Can you work these out from the model? Positions are in its coordinate system, mm. Face numbers are marked on the shaded views. A direction names the side the tool comes from. Coordinates: 2 decimals unless noted, no trailing zeros. Order: outer loops, then holes, each group sorted by start corner. A loop starts at its lowest first (then second) coordinate and runs counter-clockwise, first axis right, second up. Notation, with made-up numbers: (85, 4.25) -> (119, 4.25) arc R22 ccw to (119, 32.25) -> close; hole circle Ø11 at (78, 64). An arc over 180 degrees is marked (long way). Return JSON: item names as keys, results as strings. Group by question number.
1) If we section it at C-C, the plane y = 45.3: Please give me the cut outline in (x, z), then the cut area to 3 significant figures.
2) If we section it at B-B, the plane y = 30: Please give me the cut outline in (x, z).
3) For the marked faces 1 and 2, which set-ups out of +Z, -Z, +X, -X, +Y, -Y let a thin tool reach every point of the face, with its end or its side?
4) If we section it at A-A, the plane z = 0: Please give me the cut outline in (x, y), then the cut area to 3 significant figures.
5) If I drill on probe 1 along X at (y, z) = (0.9, -12.7); probe 2 along X at (y, z) = (29.5, -12.5), over which ranges is the centre line in solid material (lowest first)? Write a range as from..to.
6) For pin 1 (10 mm diameter, centred on x = 11.5, z = 14.5, fed in from +Y); pin 2 (6 mm diameter, centred on y = 11, z = -17.5, fed in from +X); pin 3 (12 mm diameter, centred on x = 41, y = 11.5, fed in from +Z), each with a flat end and sliding along its axis, tell me the tip position at first contact or that it passes through.
7) If we section it at D-D, the plane z = 18.25: Please give me the cut outline in (x, y).
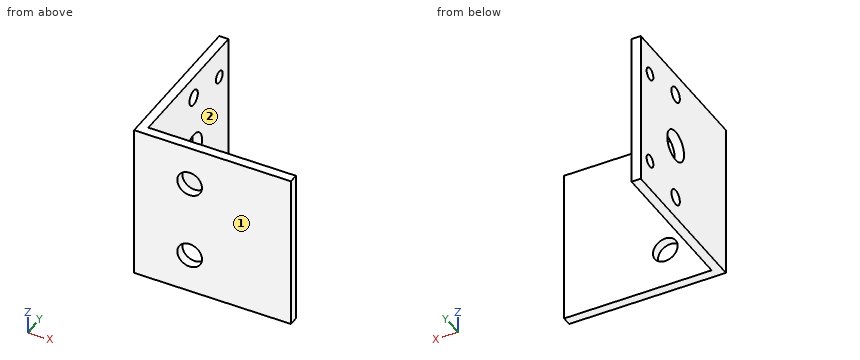
from build123d import *

# Parameters (mm, degrees)
EXTRUDE_THIN1_DEPTH = 25.4
CUT_EXTRUDE1_REACH  = 78.2
SKETCH2_R           = 2.5
SKETCH2_R_2         = 5
CUT_EXTRUDE2_REACH  = 78.2
SKETCH3_R           = 4
CUT_EXTRUDE3_REACH  = 78.2
SKETCH4_R           = 2


with BuildPart() as part:
    # Sketch1 → Extrude-Thin1 (new, symmetric)
    with BuildSketch(Plane.XY):
        Polygon((50.8, 0), (0, 0), (0, 50.8), (3, 50.8), (3, 3), (50.8, 3), align=None)
    extrude(amount=EXTRUDE_THIN1_DEPTH, both=True)

    # Sketch2 → Cut-Extrude1 (cut, up to next)
    with BuildSketch(Plane.ZY, mode=Mode.PRIVATE) as cut_extrude1_sk1:
        with Locations((-18.25, 30)):
            Circle(SKETCH2_R)
    cut_extrude1_tool1 = extrude(cut_extrude1_sk1.sketch, amount=-CUT_EXTRUDE1_REACH, mode=Mode.PRIVATE) & part.part
    # Sketch2 → Cut-Extrude1 (cut, up to next)
    with BuildSketch(Plane.ZY, mode=Mode.PRIVATE) as cut_extrude1_sk2:
        with Locations((18.25, 30)):
            Circle(SKETCH2_R)
    cut_extrude1_tool2 = extrude(cut_extrude1_sk2.sketch, amount=-CUT_EXTRUDE1_REACH, mode=Mode.PRIVATE) & part.part
    # Sketch2 → Cut-Extrude1 (cut, up to next)
    with BuildSketch(Plane.ZY, mode=Mode.PRIVATE) as cut_extrude1_sk3:
        with Locations((0, 30)):
            Circle(SKETCH2_R_2)
    cut_extrude1_tool3 = extrude(cut_extrude1_sk3.sketch, amount=-CUT_EXTRUDE1_REACH, mode=Mode.PRIVATE) & part.part
    add(cut_extrude1_tool1.solids().sort_by_distance((0, 30, -18.25))[0], mode=Mode.SUBTRACT)
    add(cut_extrude1_tool2.solids().sort_by_distance((0, 30, 18.25))[0], mode=Mode.SUBTRACT)
    add(cut_extrude1_tool3.solids().sort_by_distance((0, 30, 0))[0], mode=Mode.SUBTRACT)

    # Sketch3 → Cut-Extrude2 (cut, up to next)
    with BuildSketch(Plane.XZ, mode=Mode.PRIVATE) as cut_extrude2_sk1:
        with Locations(Location((18, 12.7, 0), (0, 0, 270))):
            Circle(SKETCH3_R)
    cut_extrude2_tool1 = extrude(cut_extrude2_sk1.sketch, amount=-CUT_EXTRUDE2_REACH, mode=Mode.PRIVATE) & part.part
    # Sketch3 → Cut-Extrude2 (cut, up to next)
    with BuildSketch(Plane.XZ, mode=Mode.PRIVATE) as cut_extrude2_sk2:
        with Locations(Location((18, -12.7, 0), (0, 0, 270))):
            Circle(SKETCH3_R)
    cut_extrude2_tool2 = extrude(cut_extrude2_sk2.sketch, amount=-CUT_EXTRUDE2_REACH, mode=Mode.PRIVATE) & part.part
    add(cut_extrude2_tool1.solids().sort_by_distance((18, 0, 12.7))[0], mode=Mode.SUBTRACT)
    add(cut_extrude2_tool2.solids().sort_by_distance((18, 0, -12.7))[0], mode=Mode.SUBTRACT)

    # Sketch4 → Cut-Extrude3 (cut, up to next)
    with BuildSketch(Plane.ZY, mode=Mode.PRIVATE) as cut_extrude3_sk1:
        with Locations((-15.5, 45.3)):
            Circle(SKETCH4_R)
    cut_extrude3_tool1 = extrude(cut_extrude3_sk1.sketch, amount=-CUT_EXTRUDE3_REACH, mode=Mode.PRIVATE) & part.part
    # Sketch4 → Cut-Extrude3 (cut, up to next)
    with BuildSketch(Plane.ZY, mode=Mode.PRIVATE) as cut_extrude3_sk2:
        with Locations((15.5, 45.3)):
            Circle(SKETCH4_R)
    cut_extrude3_tool2 = extrude(cut_extrude3_sk2.sketch, amount=-CUT_EXTRUDE3_REACH, mode=Mode.PRIVATE) & part.part
    add(cut_extrude3_tool1.solids().sort_by_distance((0, 45.3, -15.5))[0], mode=Mode.SUBTRACT)
    add(cut_extrude3_tool2.solids().sort_by_distance((0, 45.3, 15.5))[0], mode=Mode.SUBTRACT)


solid = part.part
Result sheet:
{
 "1": {"outline": "(0, -25.4) -> (3, -25.4) -> (3, -17.5) -> (0, -17.5) -> close; (0, -13.5) -> (3, -13.5) -> (3, 13.5) -> (0, 13.5) -> close; (0, 17.5) -> (3, 17.5) -> (3, 25.4) -> (0, 25.4) -> close", "area": "128 mm2"},
 "2": {"outline": "(0, -25.4) -> (3, -25.4) -> (3, -20.75) -> (0, -20.75) -> close; (0, -15.75) -> (3, -15.75) -> (3, -5) -> (0, -5) -> close; (0, 5) -> (3, 5) -> (3, 15.75) -> (0, 15.75) -> close; (0, 20.75) -> (3, 20.75) -> (3, 25.4) -> (0, 25.4) -> close"},
 "3": {"face 1": "+Z, -Z, +X, -X, -Y", "face 2": "+Z, -Z, +X, +Y"},
 "4": {"outline": "(0, 0) -> (50.8, 0) -> (50.8, 3) -> (3, 3) -> (3, 25) -> (0, 25) -> close; (0, 35) -> (3, 35) -> (3, 50.8) -> (0, 50.8) -> close", "area": "266 mm2"},
 "5": {"probe 1": "x = 0..14, 22..50.8", "probe 2": "x = 0..3"},
 "6": {"pin 1": "stops at y = 3", "pin 2": "stops at x = 3", "pin 3": "passes through"},
 "7": {"outline": "(0, 0) -> (50.8, 0) -> (50.8, 3) -> (3, 3) -> (3, 27.5) -> (0, 27.5) -> close; (0, 32.5) -> (3, 32.5) -> (3, 50.8) -> (0, 50.8) -> close"}
}
